CAD build for the part. Positions are in the model's coordinates, mm. Face numbers are marked on the shaded views. Coordinates: 2 decimals unless noted, no trailing zeros. Order: outer loops, then holes, each group sorted by start corner. A loop starts at its lowest first (then second) coordinate and runs counter-clockwise, first axis right, second up. Notation, with made-up numbers: M 0,68 L 37,68 A22 cw 37,76 Z; hole C 85,-39.5 d3. An arc over 180 degrees is marked long. Write item = value, one per line.
from build123d import *

# Parameters (mm, degrees)
SKETCH1_W                                            = 50.8
SKETCH1_H                                            = 50.8
BOSS_EXTRUDE1_DEPTH                                  = 19.05
CBORE_FOR_1_4_BINDING_HEAD_MACHINE_SCREW_D           = 6.7564
CBORE_FOR_1_4_BINDING_HEAD_MACHINE_SCREW_CBORE_D     = 14.2875
CBORE_FOR_1_4_BINDING_HEAD_MACHINE_SCREW_CBORE_DEPTH = 4.191
CBORE_FOR_2_BINDING_HEAD_MACHINE_SCREW1_D            = 2.4384
CBORE_FOR_2_BINDING_HEAD_MACHINE_SCREW1_CBORE_D      = 5.55752
CBORE_FOR_2_BINDING_HEAD_MACHINE_SCREW1_CBORE_DEPTH  = 1.27
CBORE_FOR_2_BINDING_HEAD_MACHINE_SCREW2_D            = 2.4384
CBORE_FOR_2_BINDING_HEAD_MACHINE_SCREW2_CBORE_D      = 5.55752
CBORE_FOR_2_BINDING_HEAD_MACHINE_SCREW2_CBORE_DEPTH  = 1.27


with BuildPart() as part:
    # Sketch1 → Boss-Extrude1 (new body)
    with BuildSketch(Plane(origin=(0, 0, 0), x_dir=(1, 0, 0), z_dir=(0, 1, 0))):
        Rectangle(SKETCH1_W, SKETCH1_H)
    extrude(amount=BOSS_EXTRUDE1_DEPTH)

    # CBORE for 1/4 Binding Head Machine Screw1 (through all)
    with Locations(Plane(origin=(0, 19.05, 0), x_dir=(1, 0, 0), z_dir=(0, 1, 0))):
        with Locations((0, 0)):
            CounterBoreHole(CBORE_FOR_1_4_BINDING_HEAD_MACHINE_SCREW_D / 2, CBORE_FOR_1_4_BINDING_HEAD_MACHINE_SCREW_CBORE_D / 2, CBORE_FOR_1_4_BINDING_HEAD_MACHINE_SCREW_CBORE_DEPTH)

    # CBORE for #2 Binding Head Machine Screw1 (through all)
    with Locations(Plane(origin=(0, 19.05, 0), x_dir=(1, 0, 0), z_dir=(0, 1, 0))):
        with Locations((-12.7, 12.7), (0, 0)):
            CounterBoreHole(CBORE_FOR_2_BINDING_HEAD_MACHINE_SCREW1_D / 2, CBORE_FOR_2_BINDING_HEAD_MACHINE_SCREW1_CBORE_D / 2, CBORE_FOR_2_BINDING_HEAD_MACHINE_SCREW1_CBORE_DEPTH)

    # CBORE for #2 Binding Head Machine Screw2 (through all)
    with Locations(Plane(origin=(0, 19.05, 0), x_dir=(1, 0, 0), z_dir=(0, 1, 0))):
        with Locations((12.7, 12.7), (-12.7, -12.7), (12.7, -12.7)):
            CounterBoreHole(CBORE_FOR_2_BINDING_HEAD_MACHINE_SCREW2_D / 2, CBORE_FOR_2_BINDING_HEAD_MACHINE_SCREW2_CBORE_D / 2, CBORE_FOR_2_BINDING_HEAD_MACHINE_SCREW2_CBORE_DEPTH)


solid = part.part
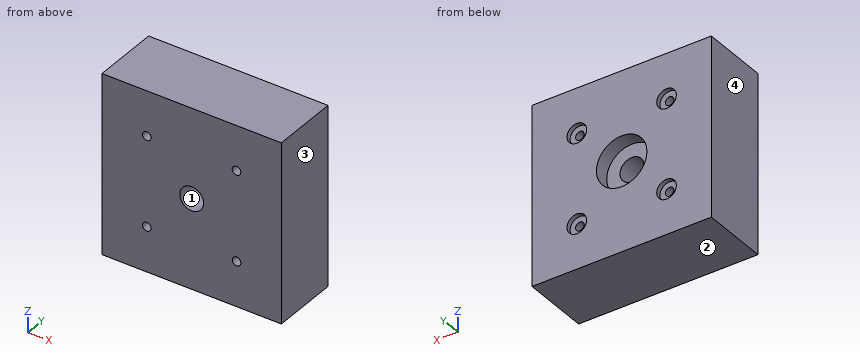
(1) Slice it at D-D, the plane z = 0. Write the cut outline in (x, y).
Evaluation:
outline = M -25.4,0 L -3.38,0 L -3.38,14.86 L -7.14,14.86 L -7.14,19.05 L -25.4,19.05 Z; M 3.38,0 L 25.4,0 L 25.4,19.05 L 7.14,19.05 L 7.14,14.86 L 3.38,14.86 Z
(2) Slice it at C-C, the plane x = 12.7. Write the cut outline in (y, z), then the cut area to 3 significant figures.
Evaluation:
outline = M 0,-25.4 L 19.05,-25.4 L 19.05,-15.48 L 17.78,-15.48 L 17.78,-13.92 L 0,-13.92 Z; M 0,-11.48 L 17.78,-11.48 L 17.78,-9.92 L 19.05,-9.92 L 19.05,9.92 L 17.78,9.92 L 17.78,11.48 L 0,11.48 Z; M 0,13.92 L 17.78,13.92 L 17.78,15.48 L 19.05,15.48 L 19.05,25.4 L 0,25.4 Z
area = 867 mm²
(3) Slice it at B-B, the plane z = 12.7. Write the cut outline in (x, y).
Evaluation:
outline = M -25.4,0 L -13.92,0 L -13.92,17.78 L -15.48,17.78 L -15.48,19.05 L -25.4,19.05 Z; M -11.48,0 L 11.48,0 L 11.48,17.78 L 9.92,17.78 L 9.92,19.05 L -9.92,19.05 L -9.92,17.78 L -11.48,17.78 Z; M 13.92,0 L 25.4,0 L 25.4,19.05 L 15.48,19.05 L 15.48,17.78 L 13.92,17.78 Z
(4) Slice it at A-A, the plane x = 0. Write the cut outline in (y, z), then the cut area to 3 significant figures.
Evaluation:
outline = M 0,-25.4 L 19.05,-25.4 L 19.05,-7.14 L 14.86,-7.14 L 14.86,-3.38 L 0,-3.38 Z; M 0,3.38 L 14.86,3.38 L 14.86,7.14 L 19.05,7.14 L 19.05,25.4 L 0,25.4 Z
area = 807 mm²
(5) Pin check, flat tip, straight feed: pin 1 Ø1.7 at (x, z) = (14, -12.5) entering from +Y. Stop position of the tip, or through.
Evaluation:
pin_1 = 17.78
(6) Wall check: line 1 (X direction, y = 11, z = -12.7); line 2 (Z direction, x = -12.7, y = 18.2). Give the ranges that are in metal, low to high. Write a range as from..to.
Evaluation:
line_1 = -25.4..-13.92, -11.48..11.48, 13.92..25.4
line_2 = -25.4..-15.48, -9.92..9.92, 15.48..25.4
(7) Pull direction X, two halves, no side cores. Call the marked faces 1, 2, 3 and 4: +X half, -X half, draft (parallel to the pull), parting line (faces both ways), or undercut.
Evaluation:
face_1 = undercut
face_2 = draft
face_3 = +X half
face_4 = -X half
